```python
from build123d import *

# Parameters (mm, degrees)
SKETCH1_W           = 152.4
SKETCH1_H           = 190.5
BOSS_EXTRUDE1_DEPTH = 88.9
BOSS_EXTRUDE2_DEPTH = 152.4


with BuildPart() as part:
    # Sketch1 → Boss-Extrude1 (new body)
    with BuildSketch(Plane(origin=(0, 0, 0), x_dir=(1, 0, 0), z_dir=(0, 1, 0))):
        with Locations((76.2, 95.25)):
            Rectangle(SKETCH1_W, SKETCH1_H)
    extrude(amount=BOSS_EXTRUDE1_DEPTH)

    # Sketch2 → Boss-Extrude2 (add)
    with BuildSketch(Plane(origin=(0, 0, 0), x_dir=(0, 0, -1), z_dir=(1, 0, 0))):
        Polygon((65.22974, 88.9), (166.82974, 88.9), (166.82974, 150.92172), (124.83338, 150.92172), (124.83338, 101.0412), (65.22974, 101.0412), align=None)
    extrude(amount=BOSS_EXTRUDE2_DEPTH)


solid = part.part
```
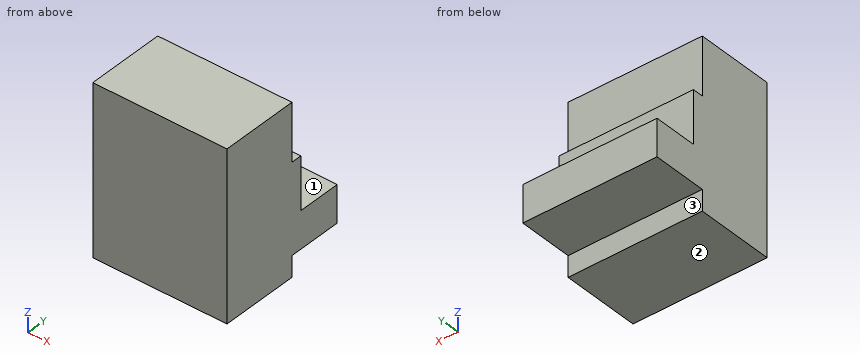
Geometry: final body of the model. Coordinates: model frame, mm. Face numbers are marked on the shaded views. A direction names the side the tool comes from. Round coordinates to 2 decimals unless told otherwise and drop trailing zeros. Order: outer loops, then holes, each group sorted by start corner. A loop starts at its lowest first (then second) coordinate and runs counter-clockwise, first axis right, second up. Notation, with made-up numbers: M -23,38.5 L 1,38.5 A21 ccw 1,75.5 Z; hole C 38.5,39 d3. An arc over 180 degrees is marked long. One line per item, written item: value.
(1) Cut plane B-B (z = -104). Return the cut outline in (x, y).
Result sheet:
outline: M 0,0 L 152.4,0 L 152.4,101.04 L 0,101.04 Z
(2) Cut plane C-C (y = 141.5). Return the cut outline in (x, z).
Result sheet:
outline: M 0,-166.83 L 152.4,-166.83 L 152.4,-124.83 L 0,-124.83 Z
(3) Line query: probe 1 along Y at (x, z) = (136, -73.5); probe 2 along Y at (x, z) = (65, -18.5); probe 3 along Z at (x, y) = (28.5, 132). Output: solid intervals per line, ascending. Write a range as [from, to].
Result sheet:
probe 1: [0, 101.04]
probe 2: [0, 88.9]
probe 3: [-166.83, -124.83]
(4) Reachability of the marked faces 1, 2 and 3 from +Z, -Z, +X, -X, +Y, -Y: full face, straight path, thin tool, end or side. Return the list, or none.
Result sheet:
face 1: +Z, +X, -X, +Y
face 2: -Z, +X, -X, +Y, -Y
face 3: -Z, +X, -X, +Y
(5) Cut plane A-A (x = 19). Return the cut outline in (y, z), and give its area (3 significant figures).
Result sheet:
outline: M 0,-190.5 L 88.9,-190.5 L 88.9,-166.83 L 150.92,-166.83 L 150.92,-124.83 L 101.04,-124.83 L 101.04,-65.23 L 88.9,-65.23 L 88.9,0 L 0,0 Z
area: 20,300 mm2
(6) Pin query (flat end, axial travel): P1, Ø5, axis at x = 103.5, z = -58.5, coming from the -Y side; P2, Ø19, axis at x = 53, z = -182, coming from the +Y side; P3, Ø25, axis at x = 53.5, y = 131.5, coming from the +Z side. Return the tip coordinate at first contact, or that it passes through.
Result sheet:
P1: y = 0
P2: y = 88.9
P3: z = -124.83
